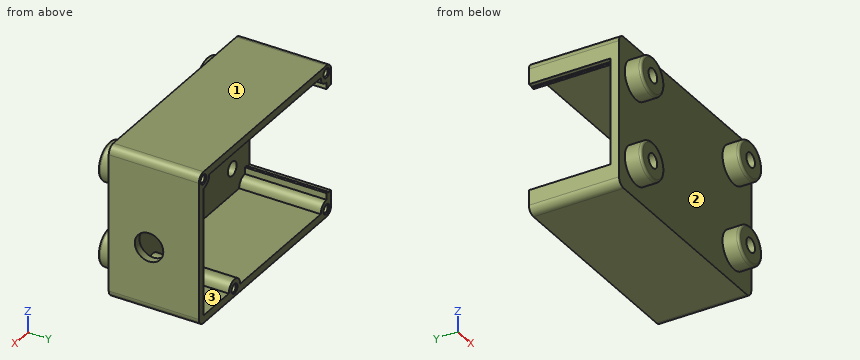
from build123d import *

# Parameters (mm, degrees)
SKETCH1_W                       = 46
SKETCH1_H                       = 32
BOSS_EXTRUDE1_DEPTH             = 19
M2X0_4_TAPPED_HOLE1_D           = 1.6
M2X0_4_TAPPED_HOLE1_DEPTH       = 6
M2X0_4_TAPPED_HOLE1_CSINK_D     = 2.05
M2X0_4_TAPPED_HOLE1_CSINK_ANGLE = 90
M2X0_4_TAPPED_HOLE1_TIP         = 0.480688495
FILLET1_R                       = 1.6
CUT_EXTRUDE3_DEPTH              = 17.2
SKETCH6_W                       = 2
SKETCH6_H                       = 22
CUT_EXTRUDE1_DEPTH              = 17.2
SKETCH7_W                       = 1
SKETCH7_H                       = 22.4
CUT_EXTRUDE2_DEPTH              = 17.2
SKETCH9_R                       = 3
CUT_EXTRUDE4_DEPTH              = 53.27810249
SKETCH10_R                      = 1.5
CUT_EXTRUDE5_DEPTH              = 10
BOSS_EXTRUDE5_START             = 3.5
SKETCH12_R                      = 4
SKETCH12_R_2                    = 1.5
BOSS_EXTRUDE5_DEPTH             = 3.5
FILLET4_R                       = 0.5


with BuildPart() as part:
    # Sketch1 → Boss-Extrude1 (new body)
    with BuildSketch(Plane(origin=(0, 0, 0), x_dir=(1, 0, 0), z_dir=(0, 1, 0))):
        with Locations((9, 0)):
            Rectangle(SKETCH1_W, SKETCH1_H)
    extrude(amount=-BOSS_EXTRUDE1_DEPTH)

    # M2x0.4 Tapped Hole1
    with Locations(Plane(origin=(0, 0, 0), x_dir=(1, 0, 0), z_dir=(0, 1, 0))):
        with Locations((-12.4, 14.4), (19.6, 14.4), (30.4, -14.4), (-12.4, -14.4)):
            CounterSinkHole(M2X0_4_TAPPED_HOLE1_D / 2, M2X0_4_TAPPED_HOLE1_CSINK_D / 2, depth=M2X0_4_TAPPED_HOLE1_DEPTH, counter_sink_angle=M2X0_4_TAPPED_HOLE1_CSINK_ANGLE)
            with Locations((0, 0, -(M2X0_4_TAPPED_HOLE1_DEPTH + M2X0_4_TAPPED_HOLE1_TIP / 2))):  # 118° drill point
                Cone(0, M2X0_4_TAPPED_HOLE1_D / 2, M2X0_4_TAPPED_HOLE1_TIP, mode=Mode.SUBTRACT)

    # Fillet1
    fillet1_edges = [part.edges().sort_by_distance(p)[0] for p in [
        (-14, -9.5, -16),
        (32, -9.5, -16),
        (32, -9.5, 16),
        (-14, -9.5, 16),
    ]]
    fillet(fillet1_edges, radius=FILLET1_R)

    # Sketch8 → Cut-Extrude3 (cut)
    with BuildSketch(Plane(origin=(0, 0, 0), x_dir=(1, 0, 0), z_dir=(0, 1, 0))):
        with BuildLine():
            Line((-10.4, 14.4), (17.6, 14.4))
            ThreePointArc((17.6, 14.4), (19.6, 12.4), (21.6, 14.4))
            Line((21.6, 14.4), (30.4, 14.4))
            Line((30.4, 14.4), (30.4, -12.4))
            ThreePointArc((30.4, -12.4), (28.985786438, -12.985786438), (28.4, -14.4))
            Line((28.4, -14.4), (-10.4, -14.4))
            ThreePointArc((-10.4, -14.4), (-10.985786438, -12.985786438), (-12.4, -12.4))
            Line((-12.4, -12.4), (-12.4, 12.4))
            ThreePointArc((-12.4, 12.4), (-10.985786438, 12.985786438), (-10.4, 14.4))
        make_face()
    extrude(amount=-CUT_EXTRUDE3_DEPTH, mode=Mode.SUBTRACT)

    # Sketch6 → Cut-Extrude1 (cut)
    with BuildSketch(Plane(origin=(0, 0, 0), x_dir=(1, 0, 0), z_dir=(0, 1, 0))):
        with Locations((-13, 0)):
            Rectangle(SKETCH6_W, SKETCH6_H)
    extrude(amount=-CUT_EXTRUDE1_DEPTH, mode=Mode.SUBTRACT)

    # Sketch7 → Cut-Extrude2 (cut)
    with BuildSketch(Plane(origin=(0, 0, 0), x_dir=(1, 0, 0), z_dir=(0, 1, 0))):
        with Locations((-13.5, 0)):
            Rectangle(SKETCH7_W, SKETCH7_H)
    extrude(amount=-CUT_EXTRUDE2_DEPTH, mode=Mode.SUBTRACT)

    # Sketch9 → Cut-Extrude4 (cut, through all)
    with BuildSketch(Plane(origin=(32, 0, 0), x_dir=(0, 0, -1), z_dir=(1, 0, 0))):
        with Locations((2.5, -10.5)):
            Circle(SKETCH9_R)
    extrude(amount=-CUT_EXTRUDE4_DEPTH, mode=Mode.SUBTRACT)

    # Sketch10 → Cut-Extrude5 (cut)
    with BuildSketch(Plane.XZ.offset(19)):
        with Locations(Location((26, 9, 0), (0, 0, 270))):
            Circle(SKETCH10_R)
        with Locations(Location((26, -9, 0), (0, 0, 90))):
            Circle(SKETCH10_R)
        with Locations(Location((-8, -9, 0), (0, 0, 270))):
            Circle(SKETCH10_R)
        with Locations(Location((-8, 9, 0), (0, 0, 90))):
            Circle(SKETCH10_R)
    extrude(amount=-CUT_EXTRUDE5_DEPTH, mode=Mode.SUBTRACT)

    # Sketch12 → Boss-Extrude5 (add)
    # profile 1 of 4: a face of its own
    with BuildSketch(Plane.XZ.offset(19).offset(BOSS_EXTRUDE5_START)):
        with Locations(Location((-8, 9, 0), (0, 0, 90))):
            Circle(SKETCH12_R)
        with Locations(Location((-8, 9, 0), (0, 0, 270))):
            Circle(SKETCH12_R_2, mode=Mode.SUBTRACT)
    # profile 2 of 4: a face of its own
    with BuildSketch(Plane.XZ.offset(19).offset(BOSS_EXTRUDE5_START)):
        with Locations(Location((26, 9, 0), (0, 0, 90))):
            Circle(SKETCH12_R)
        with Locations(Location((26, 9, 0), (0, 0, 90))):
            Circle(SKETCH12_R_2, mode=Mode.SUBTRACT)
    # profile 3 of 4: a face of its own
    with BuildSketch(Plane.XZ.offset(19).offset(BOSS_EXTRUDE5_START)):
        with Locations(Location((26, -9, 0), (0, 0, 90))):
            Circle(SKETCH12_R)
        with Locations(Location((26, -9, 0), (0, 0, 270))):
            Circle(SKETCH12_R_2, mode=Mode.SUBTRACT)
    # profile 4 of 4: a face of its own
    with BuildSketch(Plane.XZ.offset(19).offset(BOSS_EXTRUDE5_START)):
        with Locations(Location((-8, -9, 0), (0, 0, 90))):
            Circle(SKETCH12_R)
        with Locations(Location((-8, -9, 0), (0, 0, 90))):
            Circle(SKETCH12_R_2, mode=Mode.SUBTRACT)
    extrude(amount=-BOSS_EXTRUDE5_DEPTH)

    # Fillet4
    fillet4_edges = [part.edges().sort_by_distance(p)[0] for p in [
        (-8, -22.5, 5),
        (26, -22.5, 5),
        (26, -22.5, -13),
        (-8, -22.5, -13),
    ]]
    fillet(fillet4_edges, radius=FILLET4_R)


solid = part.part
Model file for the job. Use its own axes, mm. Face numbers are marked on the shaded views. A direction names the side the tool comes from. Round coordinates to 2 decimals unless told otherwise and drop trailing zeros. Loops run counter-clockwise (first coordinate to the right, second up) from the corner with the lowest first, then second, coordinate; pieces in that order, holes last. Notation, with made-up numbers: (22.5, 31.5) - (30.5, 31.5) arc R10 ccw to (30.5, 47.5) - close; hole circle Ø11 at (-24, 86). An arc over 180 degrees is marked (long way). Write each question's results on one line, items separated by ' | '.
(1) Saw through at A-A, the plane z = -9. List the corners of the cut face in (x, y), then the cut area to 3 significant figures.
Answer below:
outline: (-14, -19) - (-12, -19) - (-12, -22) arc R0.5 ccw to (-11.5, -22.5) - (-9.5, -22.5) - (-9.5, -17.2) - (-14, -17.2) - close; (-6.5, -22.5) - (-4.5, -22.5) arc R0.5 ccw to (-4, -22) - (-4, -19) - (22, -19) - (22, -22) arc R0.5 ccw to (22.5, -22.5) - (24.5, -22.5) - (24.5, -17.2) - (-6.5, -17.2) - close; (27.5, -22.5) - (29.5, -22.5) arc R0.5 ccw to (30, -22) - (30, -19) - (32, -19) - (32, 0) - (30.4, 0) - (30.4, -17.2) - (27.5, -17.2) - close | area: 134 mm^2
(2) Pin check, flat tips, straight feed: pin 1 (4 mm diameter, centred on x = 26, z = -9, fed in from +Y); pin 2 (5 mm diameter, centred on y = -10.5, z = -2.5, fed in from +X); pin 3 (1.4 mm diameter, centred on x = -12.4, z = -14.4, fed in from +Y); pin 4 (1.3 mm diameter, centred on x = -12.4, z = 14.4, fed in from -Y). Stop position of each tip, or through.
Answer below:
pin 1: stops at y = -17.2 | pin 2: passes through | pin 3: stops at y = -6.06 | pin 4: stops at y = -19
(3) 3-axis set-ups, long thin cutter, end or side, ignore diameter. For the marked faces 1, 2 and 3: which of +Z, -Z, +X, -X, +Y, -Y reach the whole face in a straight line?
Answer below:
face 1: +Z, +X, -X, +Y, -Y | face 2: -Y | face 3: +Y
(4) Wall check: L1, parallel to X at y = -17.85, z = 9; L2, parallel to X at y = -20.75, z = 9; L3, parallel to Z at x = 11, y = -17. Give the ranges that are in metal, low to high.
Answer below:
L1: x = -14 to -9.5, -6.5 to 24.5, 27.5 to 32 | L2: x = -12 to -9.5, -6.5 to -4, 22 to 24.5, 27.5 to 30 | L3: z = -16 to -14.4, 14.4 to 16
(5) Saw through at D-D, the plane y = -16.5. List the corners of the cut face in (x, z).
Answer below:
outline: (-14, -14.4) arc R1.6 ccw to (-12.4, -16) - (30.4, -16) arc R1.6 ccw to (32, -14.4) - (32, 14.4) arc R1.6 ccw to (30.4, 16) - (-12.4, 16) arc R1.6 ccw to (-14, 14.4) - (-14, 11.2) - (-13, 11.2) - (-13, 11) - (-12.4, 11) - (-12.4, 12.4) arc R2 ccw to (-10.4, 14.4) - (28.4, 14.4) arc R2 ccw to (30.4, 12.4) - (30.4, -14.4) - (21.6, -14.4) arc R2 ccw to (17.6, -14.4) - (-10.4, -14.4) arc R2 ccw to (-12.4, -12.4) - (-12.4, -11) - (-13, -11) - (-13, -11.2) - (-14, -11.2) - close
(6) Saw through at B-B, the plane y = -5.5. Count the separate pieces of the cut face and the enclosed holes in it, then the cut area to 3 significant figures.
Answer below:
separate pieces: 1 | enclosed holes: 4 | area: 209 mm^2
(7) Saw through at C-C, the plane x = 7.5. List the corners of the cut face in (y, z), then the cut area to 3 significant figures.
Answer below:
outline: (-19, -16) - (0, -16) - (0, -14.4) - (-17.2, -14.4) - (-17.2, 14.4) - (0, 14.4) - (0, 16) - (-19, 16) - close | area: 113 mm^2
